Geometry: final body of the model. Coordinates: model frame, mm. Round coordinates to 2 decimals unless told otherwise and drop trailing zeros. Loops run counter-clockwise (first coordinate to the right, second up) from the corner with the lowest first, then second, coordinate; pieces in that order, holes last. Notation, with made-up numbers: M 59.5,72.25 L 106.5,72.25 A5 ccw 106.5,81.25 Z; hole C 79.25,75.5 d4. An arc over 180 degrees is marked long. Return JSON: item names as keys, results as strings.
from build123d import *

# Parameters (mm, degrees)
SKETCH1_R           = 3.25
SKETCH1_R_2         = 3
BOSS_EXTRUDE1_DEPTH = 4.7625
FILLET3_R           = 3.18


with BuildPart() as part:
    # Sketch1 → Boss-Extrude1 (new body)
    with BuildSketch(Plane.XY):
        Polygon((27.466141976, -161.906947321), (27.466141976, -151.906947321), (42.428200405, -151.906947321), (42.428200405, -200.628730702), (67.157321136, -200.628730702), (67.157321136, -169.057449544), (107.157321136, -169.057449544), (107.157321136, -249.057449544), (-112.842678864, -249.057449544), (-112.842678864, -169.057449544), (-72.842678864, -169.057449544), (-72.842678864, -209.057449544), (27.466141976, -209.057449544), (27.466141976, -199.057449544), (29.50037366, -199.057449544), (29.50037366, -161.906947321), align=None)
        with Locations(Location((-92.842678864, -189.057449544, 0), (0, 0, 180))):
            Circle(SKETCH1_R, mode=Mode.SUBTRACT)
        with Locations(Location((87.157321136, -189.057449544, 0), (0, 0, 180))):
            Circle(SKETCH1_R, mode=Mode.SUBTRACT)
        with Locations(Location((87.157321136, -229.057449544, 0), (0, 0, 180))):
            Circle(SKETCH1_R, mode=Mode.SUBTRACT)
        with Locations(Location((-92.842678864, -229.057449544, 0), (0, 0, 180))):
            Circle(SKETCH1_R, mode=Mode.SUBTRACT)
        with Locations(Location((34.946141976, -203.976877703, 0), (0, 0, 180))):
            Circle(SKETCH1_R_2, mode=Mode.SUBTRACT)
        with Locations(Location((34.946141976, -156.986877707, 0), (0, 0, 180))):
            Circle(SKETCH1_R_2, mode=Mode.SUBTRACT)
    extrude(amount=BOSS_EXTRUDE1_DEPTH)

    # Fillet3
    fillet3_edges = [part.edges().sort_by_distance(p)[0] for p in [
        (-112.842678864, -169.057449544, 2.38125),
        (-72.842678864, -169.057449544, 2.38125),
        (-72.842678864, -209.057449544, 2.38125),
        (42.428200405, -151.906947321, 2.38125),
        (42.428200405, -200.628730702, 2.38125),
        (67.157321136, -200.628730702, 2.38125),
        (67.157321136, -169.057449544, 2.38125),
        (107.157321136, -169.057449544, 2.38125),
        (107.157321136, -249.057449544, 2.38125),
        (-112.842678864, -249.057449544, 2.38125),
    ]]
    fillet(fillet3_edges, radius=FILLET3_R)


solid = part.part
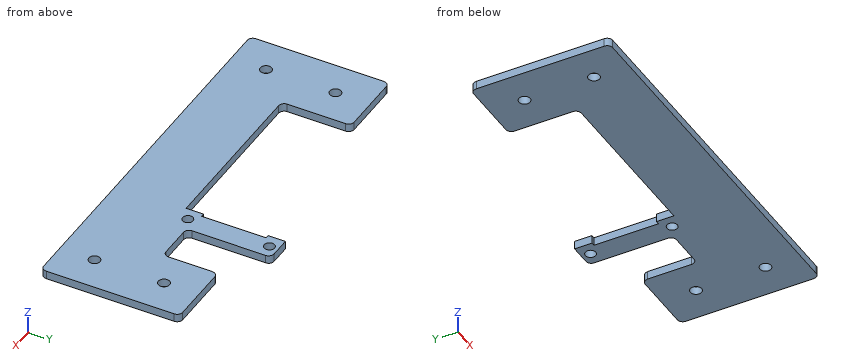
Q1. Section query C-C (y = -165). Output: boundary loops of the cut face in (x, z), plus the area to 3 significant figures.
Determined:
{"outline": "M 29.5,0 L 42.43,0 L 42.43,4.76 L 29.5,4.76 Z", "area": "61.6 mm^2"}
Q2. Pin query (flat end, axial travel): pin 1 (1 mm diameter, centred on y = -165, z = 2.5, fed in from -X); pin 2 (1.4 mm diameter, centred on x = -94.5, z = 1, fed in from +Y); pin 3 (2.5 mm diameter, centred on x = -13, z = 2.5, fed in from +Y). Return the tip coordinate at first contact, or that it passes through.
Determined:
{"pin 1": "stops at x = 29.5", "pin 2": "stops at y = -169.06", "pin 3": "stops at y = -209.06"}
Q3. Section query B-B (z = 0.85). State how many separate pieces and enclosed holes the cut face has, plus the area to 3 significant figures.
Determined:
{"separate pieces": "1", "enclosed holes": "6", "area": "12,800 mm^2"}
Q4. Section query D-D (x = -6). Output: boundary loops of the cut face in (y, z), plus the area to 4 significant figures.
Determined:
{"outline": "M -249.06,0 L -209.06,0 L -209.06,4.76 L -249.06,4.76 Z", "area": "190.5 mm^2"}
Q5. Material intervals for L1, parallel to X at y = -182.5, z = 4.6; L2, parallel to X at y = -188.5, z = 3.45; L3, parallel to Y at x = 89, z = 2.2, sorted ascending.
Determined:
{"L1": "x = -112.84 to -72.84, 29.5 to 42.43, 67.16 to 107.16", "L2": "x = -112.84 to -96.04, -89.64 to -72.84, 29.5 to 42.43, 67.16 to 83.96, 90.36 to 107.16", "L3": "y = -249.06 to -231.73, -226.38 to -191.73, -186.38 to -169.06"}
Q6. Section query A-A (y = -195). Output: boundary loops of the cut face in (x, z), plus the area to 3 significant figures.
Determined:
{"outline": "M -112.84,0 L -72.84,0 L -72.84,4.76 L -112.84,4.76 Z; M 29.5,0 L 42.43,0 L 42.43,4.76 L 29.5,4.76 Z; M 67.16,0 L 107.16,0 L 107.16,4.76 L 67.16,4.76 Z", "area": "443 mm^2"}
